The figure shows three views and two pictorial views of one solid part (mm, origin at its lowest corner). Answer the questions. A direction names the side the tool comes from. Coordinates: 2 decimals unless noted, no trailing zeros. Order: outer loops, then holes, each group sorted by start corner. A loop starts at its lowest first (then second) coordinate and runs counter-clockwise, first axis right, second up. Notation, with made-up numbers: (28, 49) - (47, 49) arc R16 ccw to (47, 57) - close; hole circle Ø11 at (-1.75, 31). An arc over 180 degrees is marked (long way). Use one line per item in the form item = value. Start each with the question number.
Item 1: Section C-C, the plane x = 10.5 is taken. Write down the section's boundary in (y, z).
Item 2: A tool of negligible diameter and unlimited length cuts with its end or side. For the marked faces 1, 2 and 3, from which of +Z, -Z, +X, -X, +Y, -Y can it reach the whole face along a straight path? Write none if from no direction.
Item 3: Section A-A, the plane z = 25 is taken. Write down the section's boundary in (x, y) (3 decimals).
Item 4: Section D-D, the plane z = 32.5 is taken. Write down the section's boundary in (x, y) (3 decimals), and give its area (3 significant figures).
Item 5: Consider line 1 along X through (y, z) = (29.5, 45.5) (3 decimals); line 2 along Y through (x, z) = (14.25, 24); line 3 along Y through (x, z) = (13.5, 19). Determine where each line is inside the solid, lowest interval first. Write a range as [from, to].
Item 6: Each of these flat-tipped pins is pushed along its axis until it touches: pin 1 Ø1.5 at (x, z) = (15.5, 24.5) entering from +Y; pin 2 Ø2 at (x, z) = (16.5, 19) entering from +Y; pin 3 Ø0.9 at (x, y) = (7, 25) entering from +Z; pin 4 Ø1 at (x, z) = (13.5, 13.5) entering from +Y. Where does it stop, or does it pass through?
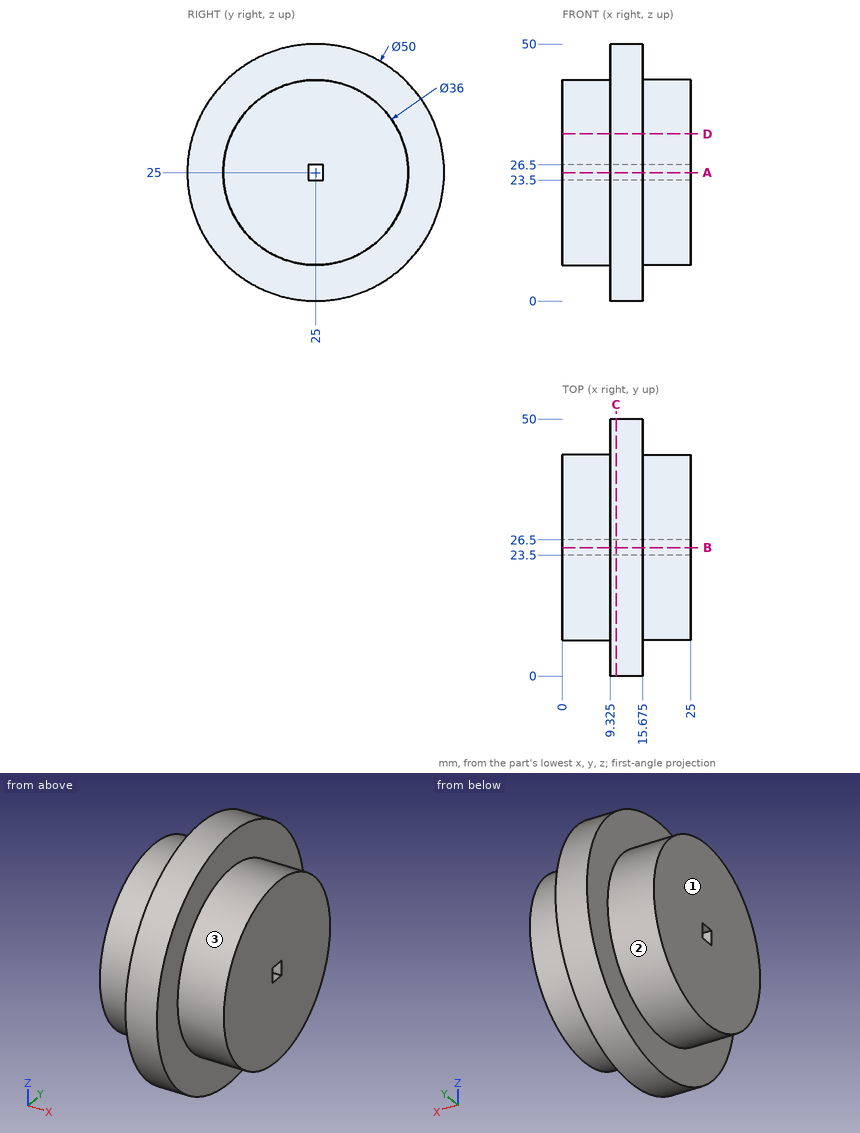
Response:
q1.outline = circle Ø50 at (25, 25); hole (23.5, 23.5) - (26.5, 23.5) - (26.5, 26.5) - (23.5, 26.5) - close
q2.face_1 = +Z, -Z, -X, +Y, -Y
q2.face_2 = -X
q2.face_3 = +X
q3.outline = (0, 7) - (9.325, 7) - (9.325, 0) - (15.675, 0) - (15.675, 7) - (25, 7) - (25, 23.5) - (0, 23.5) - close; (0, 26.5) - (25, 26.5) - (25, 43) - (15.675, 43) - (15.675, 50) - (9.325, 50) - (9.325, 43) - (0, 43) - close
q4.outline = (0, 8.637) - (9.325, 8.637) - (9.325, 1.152) - (15.675, 1.152) - (15.675, 8.637) - (25, 8.637) - (25, 41.363) - (15.675, 41.363) - (15.675, 48.848) - (9.325, 48.848) - (9.325, 41.363) - (0, 41.363) - close
q4.area = 913 mm2
q5.line_1 = [9.325, 15.675]
q5.line_2 = [0.02, 23.5], [26.5, 49.98]
q5.line_3 = [0.73, 49.27]
q6.pin_1 = 50
q6.pin_2 = 49.4
q6.pin_3 = 43
q6.pin_4 = 47.45
